Build history of the part. All positions in model axes, mm. A direction names the side the tool comes from. Round coordinates to 2 decimals unless told otherwise and drop trailing zeros. Order: outer loops, then holes, each group sorted by start corner. A loop starts at its lowest first (then second) coordinate and runs counter-clockwise, first axis right, second up. Notation, with made-up numbers: (-23.75, -34) -> (-17.75, -34) arc R9 ccw to (-17.75, -22) -> close; hole circle Ø2 at (46.25, 63). An arc over 180 degrees is marked (long way). Answer as a JSON object with one key per item and string values.
from build123d import *

# Parameters (mm, degrees)
F1_DEPTH       = 76.2
F3_D           = 15.24
F3_CBORE_D     = 40.64
F3_CBORE_DEPTH = 10.16
F4_DEPTH       = 10.16
F5_R           = 10.16
F6_DEPTH       = 76.2
F8_DEPTH       = 27.94
F9_R           = 10.16


with BuildPart() as f1:
    # F0 (on Right) → F1 (new body)
    with BuildSketch(Plane.YZ):
        Polygon((0, 35.56), (0, 0), (111.76, 0), (147.32, 35.56), (147.32, 71.12), (111.76, 71.12), (76.2, 35.56), align=None)
    extrude(amount=F1_DEPTH)

    # F3 (through all)
    with Locations(Plane.XY.offset(35.56)):
        with Locations((38.1, 40.77832)):
            CounterBoreHole(F3_D / 2, F3_CBORE_D / 2, F3_CBORE_DEPTH)

    # F2 (on face) → F4 (cut)
    with BuildSketch(Plane.XY.offset(35.56)):
        with BuildLine():
            Line((33.02, 76.2), (33.02, 60.453076))
            ThreePointArc((33.02, 60.453076), (17.78, 40.77832), (33.02, 21.103565))
            Line((33.02, 21.103565), (33.02, 0))
            Line((33.02, 0), (43.18, 0))
            Line((43.18, 0), (43.18, 21.103565))
            ThreePointArc((43.18, 21.103565), (58.42, 40.77832), (43.18, 60.453076))
            Line((43.18, 60.453076), (43.18, 76.2))
            Line((43.18, 76.2), (33.02, 76.2))
        make_face()
    extrude(amount=-F4_DEPTH, mode=Mode.SUBTRACT)

    # F5 (on face) → F6 (cut)
    with BuildSketch(Plane.YZ.offset(76.2)):
        with Locations((93.98, 20.32)):
            Circle(F5_R)
    extrude(amount=-F6_DEPTH, mode=Mode.SUBTRACT)

    # F7 (on face) → F8 (cut)
    with BuildSketch(Plane.XY.offset(71.12)):
        with BuildLine():
            Line((60.96, 137.16), (15.24, 137.16))
            ThreePointArc((15.24, 137.16), (7.62, 129.54), (15.24, 121.92))
            Line((15.24, 121.92), (60.96, 121.92))
            ThreePointArc((60.96, 121.92), (68.58, 129.54), (60.96, 137.16))
        make_face()
    extrude(amount=-F8_DEPTH, mode=Mode.SUBTRACT)

    # F9
    f9_edges = [f1.edges().sort_by_distance(p)[0] for p in [
        (0, 0, 17.78),
        (76.2, 0, 17.78),
    ]]
    fillet(f9_edges, radius=F9_R)


solid = f1.part
1) Flat gauge pins, fed straight in: pin 1 Ø12 at (y, z) = (93.98, 20.32) entering from +X; pin 2 Ø10 at (x, y) = (62.5, 57.5) entering from +Z; pin 3 Ø5 at (x, z) = (54.5, 19) entering from +Y; pin 4 Ø20.5 at (x, y) = (44.5, 43.5) entering from +Z. Where does each tip first touch, or does it go through?
Checked values:
{"pin 1": "passes through", "pin 2": "stops at z = 35.56", "pin 3": "stops at y = 133.26", "pin 4": "stops at z = 25.4"}
2) Cut at A-A, the plane x = 38.1. Give the cut face in (y, z).
Checked values:
{"outline": "(0, 0) -> (33.16, 0) -> (33.16, 25.4) -> (0, 25.4) -> close; (48.4, 0) -> (111.76, 0) -> (147.32, 35.56) -> (147.32, 71.12) -> (137.16, 71.12) -> (137.16, 43.18) -> (121.92, 43.18) -> (121.92, 71.12) -> (111.76, 71.12) -> (76.2, 35.56) -> (76.2, 25.4) -> (48.4, 25.4) -> close; hole circle Ø20.32 at (93.98, 20.32)"}
3) Cut at B-B, the plane z = 20.32. Give the cut face in (x, y).
Checked values:
{"outline": "(0, 10.16) arc R10.16 ccw to (10.16, 0) -> (66.04, 0) arc R10.16 ccw to (76.2, 10.16) -> (76.2, 83.82) -> (0, 83.82) -> close; (0, 104.14) -> (76.2, 104.14) -> (76.2, 132.08) -> (0, 132.08) -> close; hole circle Ø15.24 at (38.1, 40.78)"}
4) Cut at C-C, the plane y = 93.5. Give the cut face in (x, z), plus the area to 3 significant figures.
Checked values:
{"outline": "(0, 0) -> (76.2, 0) -> (76.2, 10.17) -> (0, 10.17) -> close; (0, 30.47) -> (76.2, 30.47) -> (76.2, 52.86) -> (0, 52.86) -> close", "area": "2,480 mm²"}
5) Cut at D-D, the plane z = 32. Give the cut face in (x, y).
Checked values:
{"outline": "(0, 10.16) arc R10.16 ccw to (10.16, 0) -> (33.02, 0) -> (33.02, 21.1) arc R20.32 cw to (33.02, 60.45) -> (33.02, 76.2) -> (43.18, 76.2) -> (43.18, 60.45) arc R20.32 cw to (43.18, 21.1) -> (43.18, 0) -> (66.04, 0) arc R10.16 ccw to (76.2, 10.16) -> (76.2, 143.76) -> (0, 143.76) -> close"}
6) Pull direction X, two halves, no side cores. Call faces 4 (the face through (38, 138, 71.12)), 5 (the face through (33.02, 11, 31)), 6 (the face through (73.145, 2.897, 17.531)): pulls with the +X half, pulls with the -X half, needs draft (parallel to the pull), parting line crosses it, or undercut.
Checked values:
{"face 4": "needs draft", "face 5": "undercut", "face 6": "pulls with the +X half"}
7) Probe L1, parallel to Y at x = 35, z = 20; L2, parallel to Y at x = 38, z = 15; L3, parallel to Z at x = 19, y = 92.5. List the from-to ranges inside material, lowest first. Write a range as from..to.
Checked values:
{"L1": "y = 0..33.82, 47.74..83.83, 104.13..131.76", "L2": "y = 0..33.16, 48.4..85.32, 102.64..126.76", "L3": "z = 0..10.27, 30.37..51.86"}
8) Which spindle directions (+Z, -Z, +X, -X, +Y, -Y) get a long thin tool onto all of the face, cutting with end or side? Do faces 1 (the face through (33.02, 68, 31)), 2 (the face through (63, 39, 35.56)), 3 (the face through (7.62, 129.71, 57.35)). Say none if no direction does.
Checked values:
{"face 1": "+Z, -Y", "face 2": "+Z, +X, -X, -Y", "face 3": "+Z"}
